from build123d import *

# Parameters (mm, degrees)
SKETCH1_R           = 32.5
BOSS_EXTRUDE1_DEPTH = 13
SKETCH2_R           = 5
CUT_EXTRUDE1_DEPTH  = 48.765049984
SKETCH3_R           = 3.808073824
CUT_EXTRUDE2_DEPTH  = 12.847377
CIRPATTERN1_START   = 0.152622896
CIRPATTERN1_DEPTH   = 12.847377104


# Read off the part's stored shape, not the designer's step: CirPattern1
with BuildPart() as part:
    # Sketch1 → Boss-Extrude1 (new body)
    with BuildSketch(Plane(origin=(0, 0, 0), x_dir=(1, 0, 0), z_dir=(0, 1, 0))):
        with Locations(Location((0, 0, 0), (0, 0, 90))):
            Circle(SKETCH1_R)
    extrude(amount=BOSS_EXTRUDE1_DEPTH)

    # Sketch2 → Cut-Extrude1 (cut, through all)
    with BuildSketch(Plane(origin=(0, 0, 0), x_dir=(1, 0, 0), z_dir=(0, 1, 0))):
        with Locations(Location((0, 0, 0), (0, 0, 90))):
            Circle(SKETCH2_R)
    extrude(amount=CUT_EXTRUDE1_DEPTH, mode=Mode.SUBTRACT)

    # Sketch3 → Cut-Extrude2 (cut)
    with BuildSketch(Plane(origin=(0, 13, 0), x_dir=(1, 0, 0), z_dir=(0, 1, 0))):
        with Locations((-4.941482649, 0)):
            Circle(SKETCH3_R)
    extrude(amount=-CUT_EXTRUDE2_DEPTH, mode=Mode.SUBTRACT)

    # CirPattern1 outline → CirPattern1 (cut)
    with BuildSketch(Plane(origin=(0, 0, 0), x_dir=(1, 0, 0), z_dir=(0, 1, 0)).offset(CIRPATTERN1_START)):
        with BuildLine():
            ThreePointArc((-3.533031177, -3.538034864), (-4.869727209, -3.807397721), (-6.215623426, -3.588591859))
            ThreePointArc((-6.215623426, -3.588591859), (-4.374778236, -7.577338177), (0, -7.177183717))
            ThreePointArc((0, -7.177183717), (4.374778236, -7.577338177), (6.215623426, -3.588591858))
            ThreePointArc((6.215623426, -3.588591858), (8.749556473, 0), (6.215623426, 3.588591858))
            ThreePointArc((6.215623426, 3.588591858), (4.374778236, 7.577338177), (0, 7.177183717))
            ThreePointArc((0, 7.177183717), (-4.374778236, 7.577338177), (-6.215623426, 3.588591858))
            ThreePointArc((-6.215623426, 3.588591858), (-4.869727209, 3.807397721), (-3.533031177, 3.538034864))
            ThreePointArc((-3.533031177, 3.538034864), (5, 0), (-3.533031177, -3.538034864))
        make_face()
    extrude(amount=CIRPATTERN1_DEPTH, mode=Mode.SUBTRACT)


solid = part.part
The model under review builds one solid part; all positions refer to its coordinate system, in mm. A direction names the side the tool comes from. Round coordinates to 2 decimals unless told otherwise and drop trailing zeros. Order: outer loops, then holes, each group sorted by start corner. A loop starts at its lowest first (then second) coordinate and runs counter-clockwise, first axis right, second up. Notation, with made-up numbers: (-15.5, -38) -> (43.5, -38) arc R9 cw to (43.5, -31) -> close; hole circle Ø2 at (-14.5, 50). An arc over 180 degrees is marked (long way). Use CSV: the item, a comma, the result in double quotes. Start each with the question number.
(1) Consider section D-D on z = 25. Write out the cut boundary in (x, y).
(2) Consider section C-C on x = -18. Write out the cut boundary in (y, z).
(3) Wall thickness on probe 1 along X at (y, z) = (0.1, 0); probe 2 along X at (y, z) = (5.75, -2); probe 3 along Z at (x, y) = (-2.5, 4): over which ranges is each line inside the solid? List them lowest first. Write a range as from..to.
(4) Mouldability with a two-part tool opening along X and no side actions: class faces 3 (the face through (-9.76, 6.41, -31)), 4 (the face through (0, 0, -7)), 5 (the face through (-8.75, 6.67, -0.07)) as pulls with the +X half, pulls with the -X half, needs draft (parallel to the pull), parting line crosses it, or undercut.
(5) Consider section B-B on y = 6. Write out the cut boundary in (x, z), and give its area (3 significant figures).
(6) Consider section A-A on z = 0. Write out the cut boundary in (x, y).
(7) Tool access review of faces 1 (the face through (4.431, 6.486, -7.544)), 2 (the face through (0, 13, 8)): name each direction out of +Z, -Z, +X, -X, +Y, -Y from which nothing blocks a thin tool from reaching the whole face with its end or side.
(8) Insertion check: pin 1 (2.5 mm diameter, centred on x = -6, z = 1, fed in from +Y); pin 2 (2 mm diameter, centred on x = -20, y = 5, fed in from -Z); pin 3 (3 mm diameter, centred on x = -22, z = 24, fed in from -Y); pin 4 (1.5 mm diameter, centred on x = 7.5, y = 7.5, fed in from +Z). Each pin has a flat end and moves straight along its axis. Give the tip position at first contact, or say it passes through.
Responses:
1,outline,"(-20.77, 0) -> (20.77, 0) -> (20.77, 13) -> (-20.77, 13) -> close"
2,outline,"(0, -27.06) -> (13, -27.06) -> (13, 27.06) -> (0, 27.06) -> close"
3,probe 1,"-32.5..-5, 5..32.5"
3,probe 2,"-32.44..-8.18, 8.18..32.44"
3,probe 3,"-32.4..-8.09, 8.09..32.4"
4,face 3,"parting line crosses it"
4,face 4,"needs draft"
4,face 5,"undercut"
5,outline,"circle Ø65 at (0, 0); hole (-6.22, -3.59) arc R3.81 ccw to (0, -7.18) arc R3.81 ccw to (6.22, -3.59) arc R3.81 ccw to (6.22, 3.59) arc R3.81 ccw to (0, 7.18) arc R3.81 ccw to (-6.22, 3.59) arc R3.81 ccw to start"
5,area,"3,100 mm²"
6,outline,"(-32.5, 0) -> (-5, 0) -> (-5, 0.15) -> (-8.75, 0.15) -> (-8.75, 13) -> (-32.5, 13) -> close; (5, 0) -> (32.5, 0) -> (32.5, 13) -> (8.75, 13) -> (8.75, 0.15) -> (5, 0.15) -> close"
7,face 1,"+Y"
7,face 2,"+Z, -Z, +X, -X, +Y"
8,pin 1,"y = 0.15"
8,pin 2,"z = -26.37"
8,pin 3,"y = 0"
8,pin 4,"z = 31.79"
